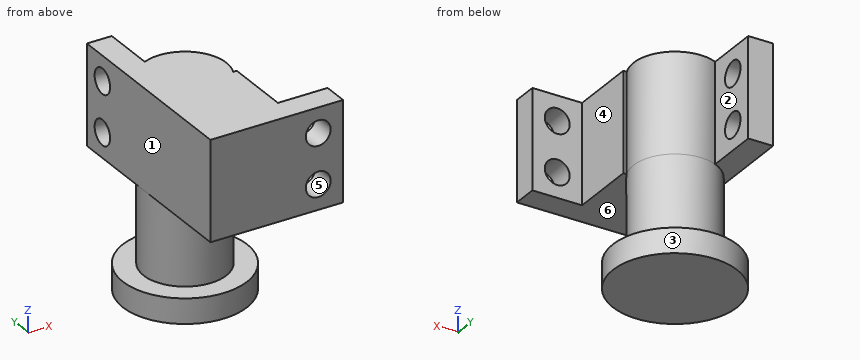
```python
from build123d import *

# Parameters (mm, degrees)
SKETCH_1_W          = 5
SKETCH_1_H          = 8
EXTRUDE_1_DEPTH     = 12
SKETCH_2_R          = 5
EXTRUDE_2_DEPTH     = 10
SKETCH_3_R          = 7.5
EXTRUDE_3_DEPTH     = 3
SKETCH_4_R          = 1.5
CUT_EXTRUDE_1_DEPTH = 3
SKETCH_5_R          = 1.5
CUT_EXTRUDE_2_DEPTH = 11
SKETCH_6_W          = 6
SKETCH_6_H          = 12
CUT_EXTRUDE_3_DEPTH = 8


with BuildPart() as part:
    # 草图1 → 凸台-拉伸1 (new body)
    with BuildSketch(Plane.XY):
        with BuildLine():
            Line((11, -2), (4.582575695, -2))
            ThreePointArc((4.582575695, -2), (3.535533906, 3.535533906), (-2, 4.582575695))
            Line((-2, 4.582575695), (-2, 11))
            Line((-2, 11), (-5, 11))
            Line((-5, 11), (-5, 0))
            Line((-5, 0), (-5, -5))
            Line((-5, -5), (0, -5))
            Line((0, -5), (11, -5))
            Line((11, -5), (11, -2))
        make_face()
        Polygon((-5, -13), (-5, -5), (0, -5), (11, -5), (11, -13), align=None)
        with Locations((-2.5, -9)):
            Rectangle(SKETCH_1_W, SKETCH_1_H)
    extrude(amount=EXTRUDE_1_DEPTH)

    # 草图2 → 凸台-拉伸2 (add)
    with BuildSketch(Plane.XY.offset(12)):
        with Locations(Location((0, 0, 0), (0, 0, 180))):
            Circle(SKETCH_2_R)
    extrude(amount=EXTRUDE_2_DEPTH)

    # 草图3 → 凸台-拉伸3 (add)
    with BuildSketch(Plane.XY.offset(22)):
        Circle(SKETCH_3_R)
    extrude(amount=EXTRUDE_3_DEPTH)

    # 草图4 → 切除-拉伸1 (cut)
    with BuildSketch(Plane(origin=(-2, 0, 0), x_dir=(0, 0, -1), z_dir=(1, 0, 0))):
        with Locations(Location((-9, 7.998538294, 0), (0, 0, 90))):
            Circle(SKETCH_4_R)
        with Locations(Location((-3, 7.998538294, 0), (0, 0, 90))):
            Circle(SKETCH_4_R)
    extrude(amount=-CUT_EXTRUDE_1_DEPTH, mode=Mode.SUBTRACT)

    # 草图5 → 切除-拉伸2 (cut)
    with BuildSketch(Plane(origin=(0, -2, 0), x_dir=(1, 0, 0), z_dir=(0, 1, 0))):
        with Locations(Location((8, -9, 0), (0, 0, 270))):
            Circle(SKETCH_5_R)
        with Locations(Location((8, -3, 0), (0, 0, 270))):
            Circle(SKETCH_5_R)
    extrude(amount=-CUT_EXTRUDE_2_DEPTH, mode=Mode.SUBTRACT)

    # 草图6 → 切除-拉伸3 (cut)
    with BuildSketch(Plane(origin=(0, -2, 0), x_dir=(1, 0, 0), z_dir=(0, 1, 0))):
        with Locations((8, -6)):
            Rectangle(SKETCH_6_W, SKETCH_6_H)
    extrude(amount=-CUT_EXTRUDE_3_DEPTH, mode=Mode.SUBTRACT)


with BuildPart() as body_2:
    # 镜向1: mirrored copy
    add(part.part.mirror(Plane.XY.offset(25)))


solid = body_2.part
```
Work out the finished part from the listing and answer in its coordinate system (mm). Face numbers are marked on the shaded views. A direction names the side the tool comes from. Coordinates: 2 decimals unless noted, no trailing zeros. Loops run counter-clockwise (first coordinate to the right, second up) from the corner with the lowest first, then second, coordinate; pieces in that order, holes last. Notation, with made-up numbers: (16, -23.5) - (59, -23.5) arc R6 cw to (59, -14.5) - close; hole circle Ø4 at (84, 53.5). An arc over 180 degrees is marked (long way). Use a Markdown table: item, result.
Item 1: Find section D-D, the plane x = 0. Determine the outline of the cut face in (y, z), and give its area (3 significant figures).
Evaluation:
| item | result |
|---|---|
| outline | (-13, 38) - (-5, 38) - (-5, 28) - (-7.5, 28) - (-7.5, 25) - (7.5, 25) - (7.5, 28) - (5, 28) - (5, 50) - (-13, 50) - close |
| area | 361 mm2 |
Item 2: For the marked faces 1, 2 and 3, determine the directions among +Z, -Z, +X, -X, +Y, -Y from which every point of the face is accessible in a straight line to the end or side of a thin tool.
Evaluation:
| item | result |
|---|---|
| face 1 | +Z, -X, +Y, -Y |
| face 2 | +Z, +Y |
| face 3 | -Z |
Item 3: Consider probe 1 along Y at (x, z) = (-4.25, 47); probe 2 along Z at (x, y) = (-1.75, 5.5); probe 3 along Y at (x, z) = (9.75, 46.25). Determine where each line is inside the solid, lowest interval first. Write a range as from..to.
Evaluation:
| item | result |
|---|---|
| probe 1 | y = -13..6.5, 9.5..11 |
| probe 2 | z = 25..28 |
| probe 3 | y = -13..-10 |
Item 4: The mould has two halves that part along X. Classify the marked faces 4, 5 and 6: +X half, -X half, draft (parallel to the pull), parting line (faces both ways), or undercut.
Evaluation:
| item | result |
|---|---|
| face 4 | +X half |
| face 5 | undercut |
| face 6 | draft |
Item 5: Find section A-A, the plane x = 8. Determine the outline of the cut face in (y, z), and give its area (3 significant figures).
Evaluation:
| item | result |
|---|---|
| outline | (-13, 38) - (-10, 38) - (-10, 39.5) - (-13, 39.5) - close; (-13, 42.5) - (-10, 42.5) - (-10, 45.5) - (-13, 45.5) - close; (-13, 48.5) - (-10, 48.5) - (-10, 50) - (-13, 50) - close |
| area | 18.0 mm2 |
Item 6: Find section C-C, the plane z = 43.75. Determine the outline of the cut face in (x, y), and give its area (3 significant figures).
Evaluation:
| item | result |
|---|---|
| outline | (-5, -13) - (11, -13) - (11, -10) - (5, -10) - (5, -2) - (4.58, -2) arc R5 ccw to (-2, 4.58) - (-2, 11) - (-5, 11) - close |
| area | 210 mm2 |
Item 7: Find section B-B, the plane z = 47. Determine the outline of the cut face in (x, y).
Evaluation:
| item | result |
|---|---|
| outline | (-5, -13) - (6.5, -13) - (6.5, -10) - (5, -10) - (5, -2) - (4.58, -2) arc R5 ccw to (-2, 4.58) - (-2, 6.5) - (-5, 6.5) - close; (-5, 9.5) - (-2, 9.5) - (-2, 11) - (-5, 11) - close; (9.5, -13) - (11, -13) - (11, -10) - (9.5, -10) - close |
Item 8: Given pin 1 Ø1.5 at (y, z) = (4.5, 41.5) entering from +X; pin 2 Ø1.8 at (x, z) = (8, 47) entering from +Y; pin 3 Ø1.5 at (y, z) = (0.5, 43.5) entering from +X; pin 4 Ø3.5 at (x, z) = (8, 41) entering from +Y, each flat-ended and moving along its own axis, determine where each tip first touches the part or whether it passes through.
Evaluation:
| item | result |
|---|---|
| pin 1 | stops at x = 3.31 |
| pin 2 | passes through |
| pin 3 | stops at x = 5 |
| pin 4 | stops at y = -10 |
